Autodesk Inventor part; units mm, degrees
ref_plane "center_point_XY" through (5, 0, 0) normal (1, 0, 0) x (0, 0, -1)
ref_plane "center_point_YZ" through (5, 0, 0) normal (0, 0, -1) x (0, 1, 0)
ref_plane "center_point_ZX" through (5, 0, 0) normal (0, 1, 0) x (1, 0, 0)
sketch "Sketch_1" plane through (0, 0, 0) normal (0, 0, 1) x (1, 0, 0)
  line L0 (10, 0) -> (0, 0)
  line L1 (0, 15.4) -> (0, 13.4)
  line L2 (0, 13.4) -> (0.433, 13.4)
  line L3 (0.433, 13.4) -> (0.433, 8.7)
  line L4 (0.433, 8.7) -> (0, 8.7)
  line L5 (0, 8.7) -> (0, 6.6)
  arc A0 (0, 6.6) -> (0.6, 6) centre (0.6, 6.6) ccw
  line L6 (0.6, 6) -> (9.4, 6)
  arc A1 (9.4, 6) -> (10, 6.6) centre (9.4, 6.6) ccw
  line L7 (10, 6.6) -> (10, 8.7)
  line L8 (10, 8.7) -> (9.567, 8.7)
  line L9 (9.567, 8.7) -> (9.567, 13.4)
  line L10 (9.567, 13.4) -> (10, 13.4)
  line L11 (10, 13.4) -> (10, 15.4)
  arc A2 (10, 15.4) -> (9.4, 16) centre (9.4, 15.4) ccw
  line L12 (9.4, 16) -> (0.6, 16)
  arc A3 (0.6, 16) -> (0, 15.4) centre (0.6, 15.4) ccw
revolve "Revolution1" add sketch "Sketch_1" angle 360 about axis through (10, 0, 0) along (1, 0, 0)
ref_plane "center_point_XY" through (5, 0, 0) normal (1, 0, 0) x (0, 0, -1)
ref_plane "center_point_YZ" through (5, 0, 0) normal (0, 0, -1) x (0, 1, 0)
ref_plane "center_point_ZX" through (5, 0, 0) normal (0, 1, 0) x (1, 0, 0)
ref_plane "to_housing_XY" through (0, 0, 0) normal (1, 0, 0) x (0, 0, -1)
ref_plane "to_housing_YZ" through (0, 0, 0) normal (0, 0, -1) x (0, 1, 0)
ref_plane "to_housing_ZX" through (0, 0, 0) normal (0, 1, 0) x (1, 0, 0)
ref_plane "to_ring_XY" through (9.134, 0, 0) normal (1, 0, 0) x (0, 0, -1)
ref_plane "to_ring_YZ" through (9.134, 0, 0) normal (0, 0, -1) x (0, 1, 0)
ref_plane "to_ring_ZX" through (9.134, 0, 0) normal (0, 1, 0) x (1, 0, 0)
properties part number "bearing_6201"
Read the model definition and answer for the solid it produces. Units are mm, in the model's axes. A direction names the side the tool comes from. Coordinates: 2 decimals unless noted, no trailing zeros. Order: outer loops, then holes, each group sorted by start corner. A loop starts at its lowest first (then second) coordinate and runs counter-clockwise, first axis right, second up. Notation, with made-up numbers: (25, 37) - (32, 37) arc R24 ccw to (32, 61) - close; hole circle Ø11 at (56.5, -17). An arc over 180 degrees is marked (long way). Use one line per item in the form item = value.
(1) Which of the six approach directions +Z, -Z, +X, -X, +Y, -Y give full straight-line access (tool end or side, diameter ignored) to faces 4 (the face through (10, -6.5, 2)), 5 (the face through (9.567, 0, -9)), 6 (the face through (0.213, -1.886, 8.493))?
Computed values:
face_4 = +Z, -Z, +X, +Y, -Y
face_5 = +X
face_6 = -X
(2) For a pull along Z with two mould halves and no side action, classify faces 1 (the face through (9.787, -13.387, 0.589)), 2 (the face through (4.94, -3.47, 15.62)), 3 (the face through (0, -1, -14)) as pulls with the +Z half, pulls with the -Z half, needs draft (parallel to the pull), parting line crosses it, or undercut.
Computed values:
face_1 = undercut
face_2 = parting line crosses it
face_3 = needs draft
(3) Given pin 1 Ø19 at (y, z) = (0, 0) entering from -X; pin 2 Ø2 at (x, z) = (4, -4) entering from -Y; pin 3 Ø2 at (x, y) = (1.5, -3.5) entering from +Z; pin 4 Ø1 at (y, z) = (-5, 11.5) entering from -X, each flat-ended and moving along its own axis, determine where each tip first touches the part or whether it passes through.
Computed values:
pin_1 = 0
pin_2 = -15.72
pin_3 = 15.8
pin_4 = 0.43
(4) Straight lines are drawn through the part: L1, parallel to Z at x = 0.35, y = 0; L2, parallel to Z at x = 9.8, y = 0; L3, parallel to Y at x = 9.25, z = 5. For each, find the intervals that lie inside material, in ascending order.
Computed values:
L1 = -15.95 to -13.4, -8.7 to -6.05, 6.05 to 8.7, 13.4 to 15.95
L2 = -15.85 to -13.4, -8.7 to -6.15, 6.15 to 8.7, 13.4 to 15.85
L3 = -15.2 to -3.32, 3.32 to 15.2
(5) Section C-C, the plane x = 1.5 is taken. Give the vertices of the cut face in (y, z), then the cut area to 3 significant figures.
Computed values:
outline = circle Ø32 at (0, 0); hole circle Ø12 at (0, 0)
area = 691 mm²
